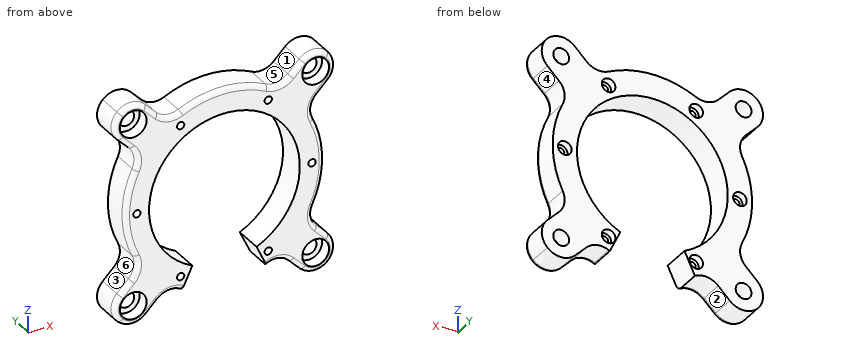
```python
from build123d import *

# Parameters (mm, degrees)
SKETCH1_R                = 41
SKETCH1_R_2              = 31
BOSS_EXTRUDE1_DEPTH      = 12
SKETCH2_R                = 1.5
CUT_EXTRUDE1_DEPTH       = 60.211485372
CIRPATTERN1_COUNT        = 6
CUT_EXTRUDE2_DEPTH       = 60.211485372
SKETCH4_R                = 2.8
CUT_EXTRUDE3_DEPTH       = 3
CIRPATTERN2_COUNT        = 6
BOSS_EXTRUDE2_DEPTH      = 12
FILLET1_R                = 8
FILLET2_R                = 8
SKETCH6_R                = 3.25
CUT_EXTRUDE4_DEPTH       = 12
SKETCH7_R                = 5.5
CUT_EXTRUDE5_DEPTH       = 5
CIRPATTERN3_COUNT        = 4
FILLET1_OF_CIRPATTERN3_R = 8
FILLET2_OF_CIRPATTERN3_R = 8
FILLET3_R                = 2


with BuildPart() as part:
    # Sketch1 → Boss-Extrude1 (new body)
    with BuildSketch(Plane(origin=(0, 0, 0), x_dir=(1, 0, 0), z_dir=(0, 1, 0))):
        with Locations(Location((0, 0, 0), (0, 0, 270))):
            Circle(SKETCH1_R)
        with Locations(Location((0, 0, 0), (0, 0, 270))):
            Circle(SKETCH1_R_2, mode=Mode.SUBTRACT)
    extrude(amount=BOSS_EXTRUDE1_DEPTH)

    # Sketch2 → Cut-Extrude1 (cut, through all)
    with BuildSketch(Plane(origin=(0, 12, 0), x_dir=(1, 0, 0), z_dir=(0, 1, 0))):
        with Locations(Location((36, 0, 0), (0, 0, 270))):
            Circle(SKETCH2_R)
    cut_extrude1 = extrude(amount=-CUT_EXTRUDE1_DEPTH, mode=Mode.SUBTRACT)

    # CirPattern1: Cut-Extrude1 ×6 about axis
    cirpattern1_axis = Axis((0, 0, 0), (0, 1, 0))
    for i in range(1, CIRPATTERN1_COUNT):
        add(cut_extrude1.rotate(cirpattern1_axis, i * 360 / CIRPATTERN1_COUNT), mode=Mode.SUBTRACT)

    # Sketch3 → Cut-Extrude2 (cut, through all)
    with BuildSketch(Plane(origin=(0, 12, 0), x_dir=(1, 0, 0), z_dir=(0, 1, 0))):
        with BuildLine():
            Line((-17.469775307, 37.091871761), (-13.2088545, 28.045073771))
            ThreePointArc((-13.2088545, 28.045073771), (0, 31), (13.2088545, 28.045073771))
            Line((13.2088545, 28.045073771), (17.469775307, 37.091871761))
            ThreePointArc((17.469775307, 37.091871761), (0, 41), (-17.469775307, 37.091871761))
        make_face()
    extrude(amount=-CUT_EXTRUDE2_DEPTH, mode=Mode.SUBTRACT)

    # Sketch4 → Cut-Extrude3 (cut)
    with BuildSketch(Plane(origin=(0, 12, 0), x_dir=(1, 0, 0), z_dir=(0, 1, 0))):
        with Locations(Location((-18, 31.176914536, 0), (0, 0, 270))):
            Circle(SKETCH4_R)
    cut_extrude3 = extrude(amount=-CUT_EXTRUDE3_DEPTH, mode=Mode.SUBTRACT)

    # CirPattern2: Cut-Extrude3 ×6 about axis
    cirpattern2_axis = Axis((0, 0, 0), (0, 1, 0))
    for i in range(1, CIRPATTERN2_COUNT):
        add(cut_extrude3.rotate(cirpattern2_axis, i * 360 / CIRPATTERN2_COUNT), mode=Mode.SUBTRACT)

    # Sketch5 → Boss-Extrude2 (add)
    with BuildSketch(Plane.XZ):
        with BuildLine():
            Line((48.81295185, 37.499243351), (43.156097601, 43.156097601))
            Line((43.156097601, 43.156097601), (37.499243351, 48.81295185))
            Line((37.499243351, 48.81295185), (22.777280167, 34.090988666))
            ThreePointArc((22.777280167, 34.090988666), (28.991378029, 28.991378029), (34.090988666, 22.777280167))
            Line((34.090988666, 22.777280167), (48.81295185, 37.499243351))
        make_face()
    boss_extrude2 = extrude(amount=-BOSS_EXTRUDE2_DEPTH)

    # Fillet1
    fillet1_edges = [part.edges().sort_by_distance(p)[0] for p in [
        (48.81295185, 6, 37.499243351),
        (37.499243351, 6, 48.81295185),
    ]]
    fillet(fillet1_edges, radius=FILLET1_R - 0.0001)  # a hair under: the kernel refuses the full size

    # Fillet2
    fillet2_edges = [part.edges().sort_by_distance(p)[0] for p in [
        (34.090988666, 6, 22.777280167),
        (22.777280167, 6, 34.090988666),
    ]]
    fillet(fillet2_edges, radius=FILLET2_R)

    # Sketch6 → Cut-Extrude4 (cut)
    with BuildSketch(Plane.XZ):
        with Locations(Location((37.499243351, 37.499243351, 0), (0, 0, 270))):
            Circle(SKETCH6_R)
    cut_extrude4 = extrude(amount=-CUT_EXTRUDE4_DEPTH, mode=Mode.SUBTRACT)

    # Sketch7 → Cut-Extrude5 (cut)
    with BuildSketch(Plane.XZ):
        with Locations(Location((37.499243351, 37.499243351, 0), (0, 0, 270))):
            Circle(SKETCH7_R)
    cut_extrude5 = extrude(amount=-CUT_EXTRUDE5_DEPTH, mode=Mode.SUBTRACT)

    # CirPattern3: Boss-Extrude2, Cut-Extrude4, Cut-Extrude5 ×4 about axis
    cirpattern3_axis = Axis((0, 0, 0), (0, 1, 0))
    add([boss_extrude2.rotate(cirpattern3_axis, i * 360 / CIRPATTERN3_COUNT) for i in range(1, CIRPATTERN3_COUNT)])
    add([cut_extrude4.rotate(cirpattern3_axis, i * 360 / CIRPATTERN3_COUNT) for i in range(1, CIRPATTERN3_COUNT)], mode=Mode.SUBTRACT)
    add([cut_extrude5.rotate(cirpattern3_axis, i * 360 / CIRPATTERN3_COUNT) for i in range(1, CIRPATTERN3_COUNT)], mode=Mode.SUBTRACT)

    # Fillet1 of CirPattern3
    fillet1_of_cirpattern3_edges = [part.edges().sort_by_distance(p)[0] for p in [
        (37.499243351, 6, -48.81295185),
        (48.81295185, 6, -37.499243351),
        (-48.81295185, 6, -37.499243351),
        (-37.499243351, 6, -48.81295185),
        (-37.499243351, 6, 48.81295185),
        (-48.81295185, 6, 37.499243351),
    ]]
    fillet(fillet1_of_cirpattern3_edges, radius=FILLET1_OF_CIRPATTERN3_R - 0.0001)  # a hair under: the kernel refuses the full size

    # Fillet2 of CirPattern3
    fillet2_of_cirpattern3_edges = [part.edges().sort_by_distance(p)[0] for p in [
        (22.777280167, 6, -34.090988666),
        (34.090988666, 6, -22.777280167),
        (-34.090988666, 6, -22.777280167),
        (-22.777280167, 6, -34.090988666),
        (-22.777280167, 6, 34.090988666),
        (-34.090988666, 6, 22.777280167),
    ]]
    fillet(fillet2_of_cirpattern3_edges, radius=FILLET2_OF_CIRPATTERN3_R)

    # Fillet3
    fillet3_edges = [part.edges().sort_by_distance(p)[0] for p in [
        (40.781034174, 0, 29.467325675),
        (29.467325675, 0, 40.781034174),
        (37.499243351, 0, 45.499284772),
        (45.499284772, 0, 37.499243351),
        (41, 0, 0),
        (36.173142632, 0, 22.75973449),
        (22.75973449, 0, 36.173142632),
        (29.467325675, 0, -40.781034174),
        (40.781034174, 0, -29.467325675),
        (45.499284772, 0, -37.499243351),
        (37.499243351, 0, -45.499284772),
        (-40.781034174, 0, -29.467325675),
        (-29.467325675, 0, -40.781034174),
        (-37.499243351, 0, -45.499284772),
        (-45.499284772, 0, -37.499243351),
        (-29.467325675, 0, 40.781034174),
        (-40.781034174, 0, 29.467325675),
        (-45.499284772, 0, 37.499243351),
        (-37.499243351, 0, 45.499284772),
        (17.703084096, 0, -36.98108724),
        (22.75973449, 0, -36.173142632),
        (36.173142632, 0, -22.75973449),
        (-41, 0, 0),
        (-36.173142632, 0, -22.75973449),
        (-22.75973449, 0, -36.173142632),
        (0, 0, 41),
        (-22.75973449, 0, 36.173142632),
        (-36.173142632, 0, 22.75973449),
        (-17.703084096, 0, -36.98108724),
    ]]
    fillet(fillet3_edges, radius=FILLET3_R)


solid = part.part
```
Model file for the job. Use its own axes, mm. Face numbers are marked on the shaded views. A direction names the side the tool comes from. Give positions to 0.01 mm unless a question says otherwise; leave off trailing zeros. Loops run counter-clockwise (first coordinate to the right, second up) from the corner with the lowest first, then second, coordinate; pieces in that order, holes last. Notation, with made-up numbers: (39.25, -32.5) -> (91.25, -32.5) arc R30 cw to (91.25, -3.5) -> close; hole circle Ø5 at (64, 35.5). An arc over 180 degrees is marked (long way). Use CSV: the item, a comma, the result in double quotes. Start each with the question number.
1) Slice it at C-C on y = 7.5. Give the number of separate pieces and of enclosed holes in the cut face, plus the area to 3 significant figures.
2) Wall check: line 1 (Z direction, x = 18, y = 9.6); line 2 (Z direction, x = -1, y = 9.25); line 3 (X direction, y = 2, z = 34). Give the ranges that are in metal, low to high.
3) Slice it at A-A on z = 0. Give the cut face in (x, y).
4) Slice it at B-B on x = 0. Give the cut face in (y, z), plus the area to 3 significant figures.
5) Mould opens along X. For the marked faces 4, 5 and 6 say: released by +X, released by -X, zero draft, split by the parting line, or undercut.
6) Tool access for the marked faces 1, 2 and 3: list every direction of +Z, -Z, +X, -X, +Y, -Y with a clear straight run to the whole face (end or side of a thin tool).
7) Flat gauge pins, fed straight in: pin 1 Ø4 at (x, z) = (18, 31.18) entering from +Y; pin 2 Ø3 at (x, y) = (-19, 9.5) entering from +Z; pin 3 Ø2.5 at (x, z) = (-36, 0) entering from -Y; pin 4 Ø3 at (x, y) = (-17.5, 4) entering from +Z. Where does each tip first touch, or does it go through?
Computed values:
1,separate pieces,"1"
1,enclosed holes,"10"
1,area,"3,010 mm^2"
2,line 1,"z = -36.84 to -33.98, -28.38 to -25.24, 25.24 to 28.38, 33.98 to 36.84"
2,line 2,"z = 30.98 to 40.99"
2,line 3,"x = -44.69 to -41.74, -33.26 to 33.26, 41.74 to 44.69"
3,outline,"(-41, 2) arc R2 ccw to (-39, 0) -> (-37.5, 0) -> (-37.5, 9) -> (-38.8, 9) -> (-38.8, 12) -> (-41, 12) -> close; (-34.5, 0) -> (-31, 0) -> (-31, 12) -> (-33.2, 12) -> (-33.2, 9) -> (-34.5, 9) -> close; (31, 0) -> (34.5, 0) -> (34.5, 9) -> (33.2, 9) -> (33.2, 12) -> (31, 12) -> close; (37.5, 0) -> (39, 0) arc R2 ccw to (41, 2) -> (41, 12) -> (38.8, 12) -> (38.8, 9) -> (37.5, 9) -> close"
4,outline,"(0, 31) -> (12, 31) -> (12, 41) -> (2, 41) arc R2 ccw to (0, 39) -> close"
4,area,"119 mm^2"
5,face 4,"released by +X"
5,face 5,"undercut"
5,face 6,"released by -X"
6,face 1,"+Z, +Y, -Y"
6,face 2,"-Z, +Y, -Y"
6,face 3,"-X, +Y, -Y"
7,pin 1,"stops at y = 9"
7,pin 2,"stops at z = 37.08"
7,pin 3,"passes through"
7,pin 4,"stops at z = 37.75"
